from build123d import *

# Parameters (mm, degrees)
SKETCH1_R           = 31.75
SKETCH1_R_2         = 14.2875
BOSS_EXTRUDE1_DEPTH = 3.175
SKETCH2_R           = 15.875
SKETCH2_R_2         = 14.2875
BOSS_EXTRUDE2_DEPTH = 25.4
SKETCH3_R           = 3.175
CUT_EXTRUDE1_DEPTH  = 25.4
BOSS_EXTRUDE3_START = 15.8496
SKETCH4_R           = 28.55968757
SKETCH4_R_2         = 15.875
SKETCH4_R_3         = 3.175
BOSS_EXTRUDE3_DEPTH = 15.8496
BOSS_EXTRUDE4_START = 15.875
BOSS_EXTRUDE4_DEPTH = 15.875
BOSS_EXTRUDE5_START = 3.175
SKETCH5_R           = 31.75
SKETCH5_R_2         = 15.875
SKETCH5_R_3         = 3.175
BOSS_EXTRUDE5_DEPTH = 3.175


with BuildPart() as part:
    # Sketch1 → Boss-Extrude1 (new body)
    with BuildSketch(Plane(origin=(0, 0, 0), x_dir=(1, 0, 0), z_dir=(0, 1, 0))):
        with Locations(Location((0, 0, 0), (0, 0, 270))):
            Circle(SKETCH1_R)
        with Locations(Location((0, 0, 0), (0, 0, 270))):
            Circle(SKETCH1_R_2, mode=Mode.SUBTRACT)
    extrude(amount=BOSS_EXTRUDE1_DEPTH)

    # Sketch2 → Boss-Extrude2 (add)
    with BuildSketch(Plane(origin=(0, 3.175, 0), x_dir=(1, 0, 0), z_dir=(0, 1, 0))):
        with Locations(Location((0, 0, 0), (0, 0, 270))):
            Circle(SKETCH2_R)
        with Locations(Location((0, 0, 0), (0, 0, 270))):
            Circle(SKETCH2_R_2, mode=Mode.SUBTRACT)
    extrude(amount=BOSS_EXTRUDE2_DEPTH)

    # Sketch3 → Cut-Extrude1 (cut)
    with BuildSketch(Plane(origin=(0, 3.175, 0), x_dir=(1, 0, 0), z_dir=(0, 1, 0))):
        with Locations(Location((-18.390705049, -13.145843594, 0), (0, 0, 270))):
            Circle(SKETCH3_R)
        with Locations(Location((-13.145843594, 18.390705049, 0), (0, 0, 270))):
            Circle(SKETCH3_R)
        with Locations(Location((18.390705049, 13.145843594, 0), (0, 0, 270))):
            Circle(SKETCH3_R)
        with Locations(Location((13.145843594, -18.390705049, 0), (0, 0, 270))):
            Circle(SKETCH3_R)
    extrude(amount=-CUT_EXTRUDE1_DEPTH, mode=Mode.SUBTRACT)

    # Sketch4 → Boss-Extrude3 (add)
    with BuildSketch(Plane(origin=(0, 3.175, 0), x_dir=(1, 0, 0), z_dir=(0, 1, 0)).offset(BOSS_EXTRUDE3_START)):
        with Locations(Location((0, 0, 0), (0, 0, 270))):
            Circle(SKETCH4_R)
        with Locations(Location((0, 0, 0), (0, 0, 270))):
            Circle(SKETCH4_R_2, mode=Mode.SUBTRACT)
        with Locations(Location((-18.390705049, -13.145843594, 0), (0, 0, 270))):
            Circle(SKETCH4_R_3, mode=Mode.SUBTRACT)
        with Locations(Location((-13.145843594, 18.390705049, 0), (0, 0, 270))):
            Circle(SKETCH4_R_3, mode=Mode.SUBTRACT)
        with Locations(Location((18.390705049, 13.145843594, 0), (0, 0, 270))):
            Circle(SKETCH4_R_3, mode=Mode.SUBTRACT)
        with Locations(Location((13.145843594, -18.390705049, 0), (0, 0, 270))):
            Circle(SKETCH4_R_3, mode=Mode.SUBTRACT)
    extrude(amount=-BOSS_EXTRUDE3_DEPTH)

    # Sketch4_9 → Boss-Extrude4 (add)
    with BuildSketch(Plane(origin=(0, 3.175, 0), x_dir=(1, 0, 0), z_dir=(0, 1, 0)).offset(BOSS_EXTRUDE4_START)):
        with BuildLine():
            ThreePointArc((27.147683603, -8.868992564), (26.798814279, -9.873160958), (26.412816089, -10.863650415))
            Line((26.412816089, -10.863650415), (28.55968757, -11.746663464))
            Line((28.55968757, -11.746663464), (29.435822625, -9.616514462))
            Line((29.435822625, -9.616514462), (27.147683603, -8.868992564))
        make_face()
        with BuildLine():
            ThreePointArc((28.518112902, -1.540451424), (28.441028918, -2.600697634), (28.324540832, -3.657340665))
            Line((28.324540832, -3.657340665), (30.626800035, -3.954614547))
            Line((30.626800035, -3.954614547), (30.921758382, -1.670288174))
            Line((30.921758382, -1.670288174), (28.518112902, -1.540451424))
        make_face()
        with BuildLine():
            ThreePointArc((27.945079936, 5.893068935), (28.145034436, 4.848998935), (28.305994926, 3.798210807))
            Line((28.305994926, 3.798210807), (30.606746691, 4.106934816))
            Line((30.606746691, 4.106934816), (30.300427406, 6.389765493))
            Line((30.300427406, 6.389765493), (27.945079936, 5.893068935))
        make_face()
        with BuildLine():
            ThreePointArc((25.467635953, 12.924986385), (25.93100237, 11.96824424), (26.358442244, 10.99492049))
            Line((26.358442244, 10.99492049), (28.500894141, 11.888603358))
            Line((28.500894141, 11.888603358), (27.614172375, 14.014367201))
            Line((27.614172375, 14.014367201), (25.467635953, 12.924986385))
        make_face()
        with BuildLine():
            ThreePointArc((21.254614667, 19.076087372), (21.949815345, 18.271873478), (22.614605282, 17.442344511))
            Line((22.614605282, 17.442344511), (24.452752754, 18.860083228))
            Line((24.452752754, 18.860083228), (23.046057132, 20.683912944))
            Line((23.046057132, 20.683912944), (21.254614667, 19.076087372))
        make_face()
        with BuildLine():
            ThreePointArc((15.593126517, 23.927184529), (16.472784678, 23.330304735), (17.329620342, 22.701101578))
            Line((17.329620342, 22.701101578), (18.738196677, 24.546279594))
            Line((18.738196677, 24.546279594), (16.907391181, 25.943884202))
            Line((16.907391181, 25.943884202), (15.593126517, 23.927184529))
        make_face()
        with BuildLine():
            Line((9.616514462, 29.435822625), (8.868992564, 27.147683603))
            ThreePointArc((8.868992564, 27.147683603), (9.873160958, 26.798814279), (10.863650415, 26.412816089))
            Line((10.863650415, 26.412816089), (11.746663464, 28.55968757))
            Line((11.746663464, 28.55968757), (9.616514462, 29.435822625))
        make_face()
        with BuildLine():
            Line((1.670288174, 30.921758382), (1.540451424, 28.518112902))
            ThreePointArc((1.540451424, 28.518112902), (2.600697634, 28.441028918), (3.657340665, 28.324540832))
            Line((3.657340665, 28.324540832), (3.954614547, 30.626800035))
            Line((3.954614547, 30.626800035), (1.670288174, 30.921758382))
        make_face()
        with BuildLine():
            Line((-6.389765493, 30.300427406), (-5.893068935, 27.945079936))
            ThreePointArc((-5.893068935, 27.945079936), (-4.848998935, 28.145034436), (-3.798210807, 28.305994926))
            Line((-3.798210807, 28.305994926), (-4.106934816, 30.606746691))
            Line((-4.106934816, 30.606746691), (-6.389765493, 30.300427406))
        make_face()
        with BuildLine():
            Line((-14.014367201, 27.614172375), (-12.924986385, 25.467635953))
            ThreePointArc((-12.924986385, 25.467635953), (-11.96824424, 25.93100237), (-10.99492049, 26.358442244))
            Line((-10.99492049, 26.358442244), (-11.888603358, 28.500894141))
            Line((-11.888603358, 28.500894141), (-14.014367201, 27.614172375))
        make_face()
        with BuildLine():
            Line((-20.683912944, 23.046057132), (-19.076087372, 21.254614667))
            ThreePointArc((-19.076087372, 21.254614667), (-18.271873478, 21.949815345), (-17.442344511, 22.614605282))
            Line((-17.442344511, 22.614605282), (-18.860083228, 24.452752754))
            Line((-18.860083228, 24.452752754), (-20.683912944, 23.046057132))
        make_face()
        with BuildLine():
            Line((-25.943884202, 16.907391181), (-23.927184529, 15.593126517))
            ThreePointArc((-23.927184529, 15.593126517), (-23.330304735, 16.472784678), (-22.701101578, 17.329620342))
            Line((-22.701101578, 17.329620342), (-24.546279594, 18.738196677))
            Line((-24.546279594, 18.738196677), (-25.943884202, 16.907391181))
        make_face()
        with BuildLine():
            Line((-29.435822625, 9.616514462), (-27.147683603, 8.868992564))
            ThreePointArc((-27.147683603, 8.868992564), (-26.798814279, 9.873160958), (-26.412816089, 10.863650415))
            Line((-26.412816089, 10.863650415), (-28.55968757, 11.746663464))
            Line((-28.55968757, 11.746663464), (-29.435822625, 9.616514462))
        make_face()
        with BuildLine():
            Line((-30.921758382, 1.670288174), (-28.518112902, 1.540451424))
            ThreePointArc((-28.518112902, 1.540451424), (-28.441028918, 2.600697634), (-28.324540832, 3.657340665))
            Line((-28.324540832, 3.657340665), (-30.626800035, 3.954614547))
            Line((-30.626800035, 3.954614547), (-30.921758382, 1.670288174))
        make_face()
        with BuildLine():
            Line((-30.300427406, -6.389765493), (-27.945079936, -5.893068935))
            ThreePointArc((-27.945079936, -5.893068935), (-28.145034436, -4.848998935), (-28.305994926, -3.798210807))
            Line((-28.305994926, -3.798210807), (-30.606746691, -4.106934816))
            Line((-30.606746691, -4.106934816), (-30.300427406, -6.389765493))
        make_face()
        with BuildLine():
            Line((-27.614172375, -14.014367201), (-25.467635953, -12.924986385))
            ThreePointArc((-25.467635953, -12.924986385), (-25.93100237, -11.96824424), (-26.358442244, -10.99492049))
            Line((-26.358442244, -10.99492049), (-28.500894141, -11.888603358))
            Line((-28.500894141, -11.888603358), (-27.614172375, -14.014367201))
        make_face()
        with BuildLine():
            Line((-23.046057132, -20.683912944), (-21.254614667, -19.076087372))
            ThreePointArc((-21.254614667, -19.076087372), (-21.949815345, -18.271873478), (-22.614605282, -17.442344511))
            Line((-22.614605282, -17.442344511), (-24.452752754, -18.860083228))
            Line((-24.452752754, -18.860083228), (-23.046057132, -20.683912944))
        make_face()
        with BuildLine():
            Line((-16.907391181, -25.943884202), (-15.593126517, -23.927184529))
            ThreePointArc((-15.593126517, -23.927184529), (-16.472784678, -23.330304735), (-17.329620342, -22.701101578))
            Line((-17.329620342, -22.701101578), (-18.738196677, -24.546279594))
            Line((-18.738196677, -24.546279594), (-16.907391181, -25.943884202))
        make_face()
        with BuildLine():
            ThreePointArc((-8.868992564, -27.147683603), (-9.873160958, -26.798814279), (-10.863650415, -26.412816089))
            Line((-10.863650415, -26.412816089), (-11.746663464, -28.55968757))
            Line((-11.746663464, -28.55968757), (-9.616514462, -29.435822625))
            Line((-9.616514462, -29.435822625), (-8.868992564, -27.147683603))
        make_face()
        with BuildLine():
            ThreePointArc((-1.540451424, -28.518112902), (-2.600697634, -28.441028918), (-3.657340665, -28.324540832))
            Line((-3.657340665, -28.324540832), (-3.954614547, -30.626800035))
            Line((-3.954614547, -30.626800035), (-1.670288174, -30.921758382))
            Line((-1.670288174, -30.921758382), (-1.540451424, -28.518112902))
        make_face()
        with BuildLine():
            ThreePointArc((5.893068935, -27.945079936), (4.848998935, -28.145034436), (3.798210807, -28.305994926))
            Line((3.798210807, -28.305994926), (4.106934816, -30.606746691))
            Line((4.106934816, -30.606746691), (6.389765493, -30.300427406))
            Line((6.389765493, -30.300427406), (5.893068935, -27.945079936))
        make_face()
        with BuildLine():
            ThreePointArc((12.924986385, -25.467635953), (11.96824424, -25.93100237), (10.99492049, -26.358442244))
            Line((10.99492049, -26.358442244), (11.888603358, -28.500894141))
            Line((11.888603358, -28.500894141), (14.014367201, -27.614172375))
            Line((14.014367201, -27.614172375), (12.924986385, -25.467635953))
        make_face()
        with BuildLine():
            ThreePointArc((23.927184529, -15.593126517), (23.330304735, -16.472784678), (22.701101578, -17.329620342))
            Line((22.701101578, -17.329620342), (24.546279594, -18.738196677))
            Line((24.546279594, -18.738196677), (25.943884202, -16.907391181))
            Line((25.943884202, -16.907391181), (23.927184529, -15.593126517))
        make_face()
        with BuildLine():
            ThreePointArc((19.076087372, -21.254614667), (18.271873478, -21.949815345), (17.442344511, -22.614605282))
            Line((17.442344511, -22.614605282), (18.860083228, -24.452752754))
            Line((18.860083228, -24.452752754), (20.683912944, -23.046057132))
            Line((20.683912944, -23.046057132), (19.076087372, -21.254614667))
        make_face()
    extrude(amount=-BOSS_EXTRUDE4_DEPTH)

    # Sketch5 → Boss-Extrude5 (add)
    with BuildSketch(Plane(origin=(0, 19.0246, 0), x_dir=(1, 0, 0), z_dir=(0, 1, 0)).offset(BOSS_EXTRUDE5_START)):
        with Locations(Location((0, 0, 0), (0, 0, 270))):
            Circle(SKETCH5_R)
        with Locations(Location((0, 0, 0), (0, 0, 270))):
            Circle(SKETCH5_R_2, mode=Mode.SUBTRACT)
        with Locations(Location((13.145843594, -18.390705049, 0), (0, 0, 270))):
            Circle(SKETCH5_R_3, mode=Mode.SUBTRACT)
        with Locations(Location((-18.390705049, -13.145843594, 0), (0, 0, 270))):
            Circle(SKETCH5_R_3, mode=Mode.SUBTRACT)
        with Locations(Location((-13.145843594, 18.390705049, 0), (0, 0, 270))):
            Circle(SKETCH5_R_3, mode=Mode.SUBTRACT)
        with Locations(Location((18.390705049, 13.145843594, 0), (0, 0, 270))):
            Circle(SKETCH5_R_3, mode=Mode.SUBTRACT)
    extrude(amount=-BOSS_EXTRUDE5_DEPTH)


solid = part.part
Work out the finished part from the listing and answer in its coordinate system (mm). A direction names the side the tool comes from. Give positions to 0.01 mm unless a question says otherwise; leave off trailing zeros. Answer in a Markdown table with one row per item.
(1) Consider L1, parallel to Y at x = 28.5, z = 4.5 (3 decimals); L2, parallel to X at y = 7.5, z = -20; L3, parallel to X at y = 10.25, z = -10.5. Determine where each line is inside the solid, lowest interval first. Write a range as [from, to].
Results list:
| item | result |
|---|---|
| L1 | y = [0, 3.175], [19.025, 22.2] |
| L2 | x = [-20.39, -15.88], [-10.41, 20.39], [22.28, 23.57] |
| L3 | x = [-29.07, -9.69], [9.69, 16.64], [20.15, 26.56] |
(2) Flat-ended cylindrical pins translate along their axes: pin 1 Ø4 at (y, z) = (17.5, 7.5) entering from +X; pin 2 Ø1.5 at (x, y) = (-3, 13.5) entering from -Z; pin 3 Ø5 at (x, z) = (18.39, -13.15) entering from -Y; pin 4 Ø5 at (y, z) = (7.5, 18) entering from +X. Find the tip coordinate at first contact, or state that the pin passes through.
Results list:
| item | result |
|---|---|
| pin 1 | stops at x = 31.14 |
| pin 2 | stops at z = -28.47 |
| pin 3 | passes through |
| pin 4 | stops at x = 25.94 |
(3) Section D-D (y = 6) is taken. State how many separate pieces and enclosed holes the cut face has, and give its area (3 significant figures).
Results list:
| item | result |
|---|---|
| separate pieces | 1 |
| enclosed holes | 5 |
| area | 1,920 mm² |
(4) A tool of negligible diameter and unlimited length cuts with its end or side. For faces 4 (the face through (29.139, 11.211, -6.145)), 5 (the face through (-1.606, 11.211, 29.737)), 6 (the face through (-1.1, 11.21, -28.54)), 7 (the face through (12.937, 11.211, 28.064)), from which of +Z, -Z, +X, -X, +Y, -Y can it reach the whole face along a straight path? Write none if from no direction.
Results list:
| item | result |
|---|---|
| face 4 | none |
| face 5 | +Z |
| face 6 | -Z |
| face 7 | +Z, +X |
(5) For a pull along X with two mould halves and no side action, classify faces 1 (the face through (19.4, 11.21, -20.96)), 2 (the face through (-30.995, 20.634, -6.883)), 3 (the face through (-28.54, 11.21, 1.1)) as pulls with the +X half, pulls with the -X half, needs draft (parallel to the pull), parting line crosses it, or undercut.
Results list:
| item | result |
|---|---|
| face 1 | undercut |
| face 2 | parting line crosses it |
| face 3 | pulls with the -X half |
